Can you work these out from the model? Positions are in its coordinate system, mm. Coordinates: 2 decimals unless noted, no trailing zeros. Loops run counter-clockwise (first coordinate to the right, second up) from the corner with the lowest first, then second, coordinate; pieces in that order, holes last. Notation, with made-up numbers: (-17.75, -31.75) -> (-0.75, -31.75) arc R5 ccw to (-0.75, -22.75) -> close; hole circle Ø4 at (58.5, -18). An arc over 180 degrees is marked (long way). Put each result on its own line as item: value. Start each with the question number.
Item 1: If we section it at B-B on x = 4.75: Please give me the cut outline in (y, z).
Item 2: If we section it at A-A on y = -12.5: Please give me the cut outline in (x, z).
Item 3: We'd pull the mould along X, two halves only. Please class faces 1 (the conical face through (-2.233, -13.98, -2.912)), 2 (the cylindrical face through (-5.37, -12.68, -1.19)), 3 (the flat face through (-2, -25, -4)): pulls with the +X half, pulls with the -X half, needs draft (parallel to the pull), parting line crosses it, or undercut.
Item 4: Please list where these lines run through material, in increasing order: L1, parallel to Z at x = 1.75, y = -8; L2, parallel to Z at x = 3.25, y = -22.75; L3, parallel to X at y = -15.75, z = -2.25. Write a range as from..to.
Item 5: If we section it at C-C on y = -2: Please give me the cut outline in (x, z) (1 decimal).
Item 6: Will these pins go through, and if not, where does the flat tip stop? P1, Ø1.4, axis at x = 0, z = 0, coming from the -Y side; P2, Ø1.5, axis at y = -7, z = -3, coming from the +X side; P3, Ø1.5, axis at y = -4.5, z = 3, coming from the -X side.
```python
from build123d import *


with BuildPart() as f1:
    # F0 (on Right) → F1 (revolve)
    with BuildSketch(Plane.YZ):
        with BuildLine():
            Line((-0.031651, 0.875), (0, 0.875))
            Line((0, 0.875), (0, 5.5))
            Line((0, 5.5), (-25, 5.5))
            Line((-25, 5.5), (-25, 4))
            Line((-25, 4), (-3.26508, 3.347329))
            Line((-3.26508, 3.347329), (-1.204977, 1.499324))
            ThreePointArc((-1.204977, 1.499324), (-0.545392, 1.324208), (-0.031651, 0.875))
        make_face()
    revolve(axis=Axis((0, -12.5, 0), (0, 1, 0)))


solid = f1.part
```
Solutions:
1. outline: (-25, -2.77) -> (0, -2.77) -> (0, 2.77) -> (-25, 2.77) -> close
2. outline: circle Ø11 at (0, 0); hole circle Ø7.25 at (0, 0)
3. face 1: undercut
3. face 2: parting line crosses it
3. face 3: needs draft
4. L1: -5.21..-3.02, 3.02..5.21
4. L2: -4.44..-2.21, 2.21..4.44
4. L3: -5.02..-2.97, 2.97..5.02
5. outline: circle Ø11 at (0, 0); hole circle Ø4.4 at (0, 0)
6. P1: through
6. P2: x = 5.02
6. P3: x = -5.02
